```python
from build123d import *

# Parameters (mm, degrees)
EXTRUDE1_DEPTH     = 48.26
SKETCH3_OUTSIDE_W  = 133.914
SKETCH3_OUTSIDE_H  = 80.574
CUT_EXTRUDE1_DEPTH = 127
FILLET1_R          = 12.7
FILLET2_R          = 12.7
SKETCH8_W          = 20
SKETCH8_H          = 10
CUT_EXTRUDE2_DEPTH = 12.7


with BuildPart() as part:
    # Sketch1 → Extrude1 (new body)
    with BuildSketch(Plane(origin=(0, 0, 0), x_dir=(1, 0, 0), z_dir=(0, 1, 0))):
        Polygon((-44.45, 101.6), (44.45, 101.6), (44.45, 57.94375), (57.15, 50.8), (28.575, 0), (-28.575, 0), (-44.45, 50.8), align=None)
    extrude(amount=EXTRUDE1_DEPTH)

    # Sketch3 outside → Cut-Extrude1 (cut, symmetric)
    with BuildSketch(Plane.ZY.offset(44.45)):
        with Locations((-50.8, 24.13)):
            Rectangle(SKETCH3_OUTSIDE_W, SKETCH3_OUTSIDE_H)
        Polygon((0, 41.445288221), (-101.6, 48.26), (-101.6, 22.86), (-68.397585835, 20.632983436), (-57.94375, 9.084619968), (-25.4, 0), (0, 5.240594668), align=None, mode=Mode.SUBTRACT)
    extrude(amount=CUT_EXTRUDE1_DEPTH, both=True, mode=Mode.SUBTRACT)

    # Fillet1
    fillet1_edges = [part.edges().sort_by_distance(p)[0] for p in [
        (-44.45, 35.56, -101.6),
        (44.45, 35.56, -101.6),
        (0, 48.26, -101.6),
        (-44.45, 46.556322055, -76.2),
        (-36.5125, 43.148966165, -25.4),
        (42.8625, 43.148966165, -25.4),
        (50.8, 45.092223821, -54.371875),
        (44.45, 46.795901766, -79.771875),
    ]]
    fillet(fillet1_edges, radius=FILLET1_R)

    # Fillet2
    fillet2_edges = [part.edges().sort_by_distance(p)[0] for p in [
        (-40.48125, 3.545217548, -38.1),
        (-32.54375, 2.620297334, -12.7),
        (50.00625, 3.545217548, -38.1),
        (35.71875, 2.620297334, -12.7),
    ]]
    fillet(fillet2_edges, radius=FILLET2_R)

    # Sketch8 → Cut-Extrude2 (cut)
    with BuildSketch(Plane.XY):
        with Locations((0.104168421, 23.306375587)):
            Rectangle(SKETCH8_W, SKETCH8_H)
    extrude(amount=-CUT_EXTRUDE2_DEPTH, mode=Mode.SUBTRACT)


solid = part.part
```
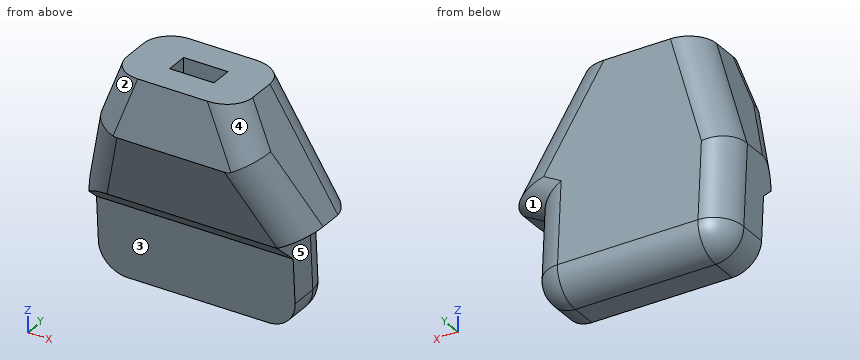
For this review, take the finished solid that the model builds, in its own axes (mm). Face numbers are marked on the shaded views. A direction names the side the tool comes from. Coordinates: 2 decimals unless noted, no trailing zeros. Loops run counter-clockwise (first coordinate to the right, second up) from the corner with the lowest first, then second, coordinate; pieces in that order, holes last. Notation, with made-up numbers: (63, 80) - (78, 80) arc R21 cw to (78, 105) - close; hole circle Ø4 at (14, 1.5). An arc over 180 degrees is marked (long way). Use one line per item in the form item = value. Start each with the question number.
1) To check wall thickness, follow probe 1 along X at (y, z) = (33, -75.5); probe 2 along Y at (x, z) = (6.5, -11). State the ranges of each line that lie inside material, in increasing order. Write a range as from..to.
2) For the marked faces 4 and 5, list the 3-axis set-ups (+Z, -Z, +X, -X, +Y, -Y) from which the entire face can be reached by the end or side of a thin tool; tool diameter is ignored.
3) Take a section at B-B (x = -12). State the section outline as (y, z) points, plus the area to 3 significant figures.
4) Take a section at A-A (x = 0). State the section outline as (y, z) points, plus the area to 3 significant figures.
5) For pin 1 (2 mm diameter, centred on x = 45.5, z = -44.5, fed in from -Y); pin 2 (10 mm diameter, centred on x = -10.5, z = -70, fed in from -Y); pin 3 (4 mm diameter, centred on x = -1.5, z = -7, fed in from +Y), all flat-tipped, find the tip position at first contact; note any pin that passes through.
6) Draft analysis for pull direction Z (two halves, no side actions). For the marked faces 1, 2 and 3, state which applies: released by +Z, released by -Z, zero draft, split by the parting line, or undercut.
From the geometry:
q1.probe_1 = -44.45..44.45
q1.probe_2 = 2.97..18.31, 28.31..42.18
q2.face_4 = +Z, +X, -Y
q2.face_5 = -Z, +X, +Y, -Y
q3.outline = (0, -25.4) - (9.08, -57.94) - (20.63, -68.4) - (22.86, -101.6) - (34.68, -101.6) arc R12.7 ccw to (47.35, -88.05) - (41.45, 0) - (5.24, 0) - close
q3.area = 3,420 mm2
q4.outline = (0, -25.4) - (9.08, -57.94) - (20.63, -68.4) - (22.86, -101.6) - (34.68, -101.6) arc R12.7 ccw to (47.35, -88.05) - (41.45, 0) - (28.31, 0) - (28.31, -12.7) - (18.31, -12.7) - (18.31, 0) - (5.24, 0) - close
q4.area = 3,300 mm2
q5.pin_1 = 7.05
q5.pin_2 = 16.88
q5.pin_3 = 42.05
q6.face_1 = undercut
q6.face_2 = released by +Z
q6.face_3 = released by -Z
